Solid Edge part; units mm, degrees
sketch "Sketch1" plane through (0, 0, 0) normal (0, -1, 0) x (1, 0, 0)
  line L0 (-14, -12) -> (14, -12)
  line L1 (14, -12) -> (14, 12)
  line L2 (14, 12) -> (-14, 12)
  line L3 (-14, 12) -> (-14, -12)
  dimension "D1" = 14
  dimension "D2" = 14
extrude "Protrusion1" add sketch "Sketch1" along normal mid plane 5
sketch "Sketch2" plane through (0, -2.5, 0) normal (0, -1, 0) x (1, 0, 0)
  circle A0 centre (0, 12) radius 12
extrude "Extrusionsausschnitt_1" cut sketch "Sketch2" against normal blind 221
hole "Bohrung_1" at (-10, 0, -12) direction (0, 0, 1) diameter 3.5 depth 8
hole "Hole1" at (10, 0, -12) direction (0, 0, 1) diameter 3.5 depth 8
mirror "Mirror1" about plane through (-13.5, 0, 12) normal (0, 0, 1) of "Protrusion1", "Extrusionsausschnitt_1", "Bohrung_1", "Hole1"
properties material "Aluminiumlegierung:3.0205, Al 99.0, EN-AW 1200"
Build history of the part. All positions in model axes, mm. A direction names the side the tool comes from. Round coordinates to 2 decimals unless told otherwise and drop trailing zeros. Loops run counter-clockwise (first coordinate to the right, second up) from the corner with the lowest first, then second, coordinate; pieces in that order, holes last. Notation, with made-up numbers: (18.5, 44.5) -> (42.5, 44.5) arc R16 ccw to (42.5, 66.5) -> close; hole circle Ø4 at (25.5, 49). An arc over 180 degrees is marked (long way). One line per item, written item: value. Start each with the question number.
Q1. Probe line 1 along X through (y, z) = (0.05, 31.5); line 2 along Z through (x, y) = (0, 0); line 3 along X through (y, z) = (1.6, 33). List the from-to ranges inside material, lowest first.
Q2. Two-plate mould, pull along X, no slides. Class faces 1 (the face through (14, 0, 12)), 2 (the face through (6, 2.5, 23)), 3 (the face through (-10, 0, -4)): released by +X, released by -X, zero draft, split by the parting line, or undercut.
Q3. Cut at B-B on x = 0. List the corners of the cut face in (y, z).
Q4. Cut at A-A on z = 12. List the corners of the cut face in (x, y), plus the area to 3 significant figures.
Q5. Cut at D-D on y = 0. List the corners of the cut face in (x, z), plus the area to 3 significant figures.
Q6. Cut at C-C on z = -8.5. List the corners of the cut face in (x, y).
Q7. Drop flat-ended pins along their axis: pin 1 Ø2 at (x, y) = (10, 0) entering from -Z; pin 2 Ø1 at (x, y) = (-9.5, 0.5) entering from +Z. Give the stop position or say it passes through.
Q8. 3-axis set-ups, long thin cutter, end or side, ignore diameter. For faces 4 (the face through (0, 0, 36)), 5 (the face through (-10, 0, 28)), 6 (the face through (-11.735, -0.228, -7.944)): which of +Z, -Z, +X, -X, +Y, -Y reach the whole face in a straight line?
Computed:
1. line 1: -14 to -11.75, -8.25 to 8.25, 11.75 to 14
1. line 2: -12 to 0, 24 to 36
1. line 3: -14 to -10.71, -9.29 to 9.29, 10.71 to 14
2. face 1: released by +X
2. face 2: zero draft
2. face 3: undercut
3. outline: (-2.5, -12) -> (2.5, -12) -> (2.5, 0) -> (-2.5, 0) -> close; (-2.5, 24) -> (2.5, 24) -> (2.5, 36) -> (-2.5, 36) -> close
4. outline: (-14, -2.5) -> (-12, -2.5) -> (-12, 2.5) -> (-14, 2.5) -> close; (12, -2.5) -> (14, -2.5) -> (14, 2.5) -> (12, 2.5) -> close
4. area: 20.0 mm²
5. outline: (-14, -12) -> (-11.75, -12) -> (-11.75, -4) -> (-8.25, -4) -> (-8.25, -12) -> (8.25, -12) -> (8.25, -4) -> (11.75, -4) -> (11.75, -12) -> (14, -12) -> (14, 36) -> (11.75, 36) -> (11.75, 28) -> (8.25, 28) -> (8.25, 36) -> (-8.25, 36) -> (-8.25, 28) -> (-11.75, 28) -> (-11.75, 36) -> (-14, 36) -> close; hole circle Ø24 at (0, 12)
5. area: 780 mm²
6. outline: (-14, -2.5) -> (14, -2.5) -> (14, 2.5) -> (-14, 2.5) -> close; hole circle Ø3.5 at (-10, 0); hole circle Ø3.5 at (10, 0)
7. pin 1: z = -4
7. pin 2: z = 28
8. face 4: +Z, +X, -X, +Y, -Y
8. face 5: +Z
8. face 6: -Z
